Here's how the part is built. I have some questions about the finished solid (model axes, mm). Coordinates: 2 decimals unless noted, no trailing zeros. Write each loop counter-clockwise with the first axis right and the second up, starting at its lowest first coordinate (ties: lowest second). Pieces come first, ordered by that corner, then holes.
(1) Please list where these lines run through material, in increasing order: probe 1 along Y at (x, z) = (0, 5.8) (3 decimals); probe 2 along Y at (x, z) = (0, -5.7) (3 decimals); probe 3 along X at (y, z) = (-115, 0.5).
(2) Imagine slicing it at B-B, the plane y = 75. List the corners of the cut face in (x, z) for me (1 decimal), plus the area to 3 significant figures.
(3) For pin 1 Ø2.5 at (x, y) = (0, 100) entering from -Z; pin 2 Ø1 at (y, z) = (-126.5, 4.5) entering from +X; pin 3 Ø3 at (y, z) = (-10, -4.5) entering from +X; pin 4 Ø6 at (y, z) = (132, 4) entering from +X, each with a flat end and sliding along its axis, tell me the tip position at first contact or that it passes through.
(4) Imagine slicing it at A-A, the plane z = 0. List the corners of the cut face in (x, y) for me (1 decimal), plus the area to 3 significant figures.
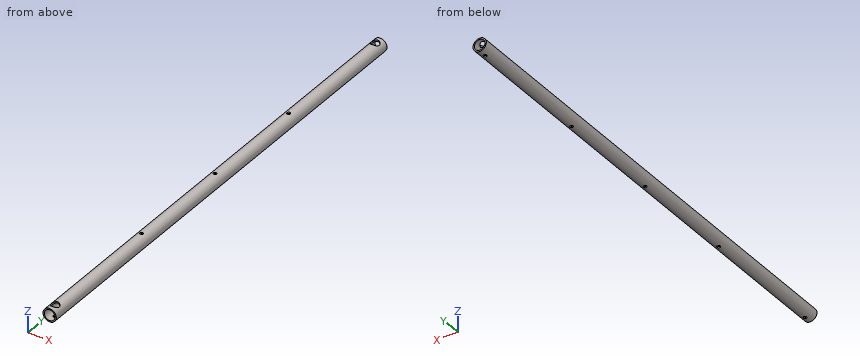
```python
from build123d import *

# Parameters (mm, degrees)
SKETCH_R         = 6.095
SKETCH_R_2       = 4.8895
PAD_DEPTH        = 225
HOLE_D           = 3.05
HOLE_DEPTH       = 25
HOLE_CBORE_D     = 7.62
HOLE_CBORE_DEPTH = 5
SKETCH002_R      = 1.525
HOLE001_DEPTH    = 25


with BuildPart() as part:
    # Sketch → Pad (new body, symmetric)
    with BuildSketch(Plane.XZ):
        Circle(SKETCH_R)
        Circle(SKETCH_R_2, mode=Mode.SUBTRACT)
    extrude(amount=PAD_DEPTH, both=True)

    # Hole
    with Locations(Plane.XY.offset(7)):
        with Locations((0, -217.79), (0, 217.79)):
            CounterBoreHole(HOLE_D / 2, HOLE_CBORE_D / 2, HOLE_CBORE_DEPTH, depth=HOLE_DEPTH)

    # Sketch002 → Hole001 (cut)
    with BuildSketch(Plane.XY.offset(7)):
        Circle(SKETCH002_R)
        with Locations((0, -100)):
            Circle(SKETCH002_R)
        with Locations((0, 100)):
            Circle(SKETCH002_R)
    extrude(amount=-HOLE001_DEPTH, mode=Mode.SUBTRACT)


solid = part.part
```
Recorded:
1. probe 1: y = -225 to -221.6, -213.98 to -101.525, -98.475 to -1.525, 1.525 to 98.475, 101.525 to 213.98, 221.6 to 225
1. probe 2: y = -225 to -219.315, -216.265 to -101.525, -98.475 to -1.525, 1.525 to 98.475, 101.525 to 216.265, 219.315 to 225
1. probe 3: x = -6.07 to -4.86, 4.86 to 6.07
2. outline: circle Ø12.2 at (0, 0); hole circle Ø9.8 at (0, 0)
2. area: 41.6 mm2
3. pin 1: passes through
3. pin 2: stops at x = 4.6
3. pin 3: stops at x = 5.31
3. pin 4: stops at x = 6.01
4. outline: (-6.1, -225) - (-4.9, -225) - (-4.9, 225) - (-6.1, 225) - close; (4.9, -225) - (6.1, -225) - (6.1, 225) - (4.9, 225) - close
4. area: 1,080 mm2
